Geometry check sheet. Reference: drawing and pictorial views, mm from the part's lowest x, y, z. Round coordinates to 2 decimals unless told otherwise and drop trailing zeros. Loops run counter-clockwise (first coordinate to the right, second up) from the corner with the lowest first, then second, coordinate; pieces in that order, holes last. Notation, with made-up numbers: (37, 39) - (72, 39) arc R22 cw to (72, 78) - close; hole circle Ø8 at (-18, 17.25). An arc over 180 degrees is marked (long way). Put each result on its own line as item: value. Start each with the question number.
Item 1: Gauge pin test, flat ends, axial feed: pin 1 Ø1.5 at (x, z) = (6, 30.5) entering from +Y (3 decimals); pin 2 Ø6 at (y, z) = (26, 18) entering from -X. Record the tip position at first contact, or that the pin passes through.
Item 2: Section check B-B, the plane x = 2. Record the cut outline in (y, z).
Item 3: Material ranges on line 1 along Y through (x, z) = (10.75, 10); line 2 along Z through (x, y) = (7.5, 9); line 3 along Z through (x, y) = (12.5, 11.5), recorded low to high.
Item 4: Section check D-D, the plane y = 12. Record the cut outline in (x, z), and give its area (3 significant figures).
Item 5: Section check C-C, the plane z = 30. Record the cut outline in (x, y).
Item 6: Section check A-A, the plane y = 4. Record the cut outline in (x, z).
Item 7: Draft check along Z on the marked faces 1, 2, 3 and 4. Enter one of: pulls with the +Z half, pulls with the -Z half, needs draft (parallel to the pull), parting line crosses it, or undercut.
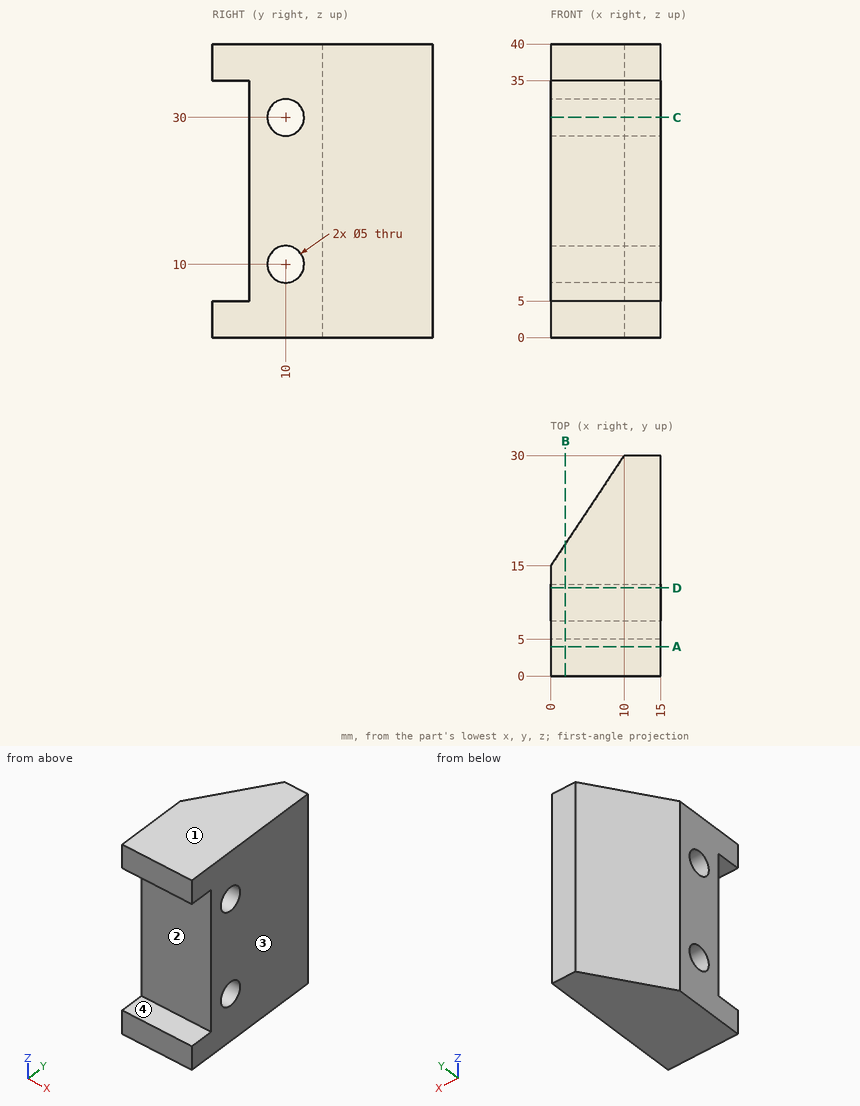
Check result:
1. pin 1: y = 25.125
1. pin 2: x = 5.33
2. outline: (0, 0) - (18, 0) - (18, 40) - (0, 40) - (0, 35) - (5, 35) - (5, 5) - (0, 5) - close; hole circle Ø5 at (10, 10); hole circle Ø5 at (10, 30)
3. line 1: 5 to 7.5, 12.5 to 30
3. line 2: 0 to 7.71, 12.29 to 27.71, 32.29 to 40
3. line 3: 0 to 8, 12 to 28, 32 to 40
4. outline: (0, 0) - (15, 0) - (15, 8.5) - (0, 8.5) - close; (0, 11.5) - (15, 11.5) - (15, 28.5) - (0, 28.5) - close; (0, 31.5) - (15, 31.5) - (15, 40) - (0, 40) - close
4. area: 510 mm²
5. outline: (0, 5) - (15, 5) - (15, 7.5) - (0, 7.5) - close; (0, 12.5) - (15, 12.5) - (15, 30) - (10, 30) - (0, 15) - close
6. outline: (0, 0) - (15, 0) - (15, 5) - (0, 5) - close; (0, 35) - (15, 35) - (15, 40) - (0, 40) - close
7. face 1: pulls with the +Z half
7. face 2: undercut
7. face 3: needs draft
7. face 4: undercut
